```python
from build123d import *

# Parameters (mm, degrees)
F0_W     = 22.349994
F0_H     = 28.762516
F0_R     = 8
F0_R_2   = 2.2479
F1_DEPTH = 3.175
F2_W     = 22.349994
F2_H     = 20.825016
F2_R     = 8
F3_DEPTH = 1.82499
F4_W     = 22.349994
F4_H     = 20.825016
F4_R     = 8
F4_R_2   = 6.412497
F5_DEPTH = 1.5875
F6_R     = 3.96875


with BuildPart() as f1:
    # F0 (on Top) → F1 (new body)
    with BuildSketch(Plane.XY):
        with Locations((0, 14.381258)):
            Rectangle(F0_W, F0_H)
        with Locations((0, 9.650006)):
            Circle(F0_R, mode=Mode.SUBTRACT)
        with Locations((-7.206247, 24.793766)):
            Circle(F0_R_2, mode=Mode.SUBTRACT)
        with Locations((7.206247, 24.793766)):
            Circle(F0_R_2, mode=Mode.SUBTRACT)
    extrude(amount=F1_DEPTH)

    # F2 (on face) → F3 (join)
    with BuildSketch(Plane.XY.offset(3.175)):
        with Locations((0, 10.412508)):
            Rectangle(F2_W, F2_H)
        with Locations((0, 9.650006)):
            Circle(F2_R, mode=Mode.SUBTRACT)
    extrude(amount=F3_DEPTH)

    # F4 (on face) → F5 (join)
    with BuildSketch(Plane.XY.offset(4.99999)):
        with Locations((0, 10.412508)):
            Rectangle(F4_W, F4_H)
        with Locations((0, 9.650006)):
            Circle(F4_R, mode=Mode.SUBTRACT)
        with Locations((0, 9.650006)):
            Circle(F4_R)
        with Locations((0, 9.650006)):
            Circle(F4_R_2, mode=Mode.SUBTRACT)
    extrude(amount=F5_DEPTH)

    # F6
    f6_edges = [f1.edges().sort_by_distance(p)[0] for p in [
        (-11.174997, 28.762516, 1.5875),
    ]]
    fillet(f6_edges, radius=F6_R)


solid = f1.part
```
Check sheet for the modelled part. Datum: model origin and axes. Units: mm. A direction names the side the tool comes from. Give positions to 0.01 mm unless a question says otherwise; leave off trailing zeros. Write each loop counter-clockwise with the first axis right and the second up, starting at its lowest first coordinate (ties: lowest second). Pieces come first, ordered by that corner, then holes. Notation, with made-up numbers: (-4.5, -9) - (-0.5, -9) arc R25 ccw to (-0.5, 29) - close; hole circle Ø4 at (-5, 68). An arc over 180 degrees is marked (long way). Answer as a JSON object with one key per item and string values. Group by question number.
1) Sectioned sample at C-C (z = 1). Give the number of separate pieces and of enclosed holes in the cut face, then the cut area to 3 significant figures.
2) Sectioned sample at B-B (z = 4.5). Record the cut outline in (x, y) (3 decimals), then the cut area to 3 significant figures.
3) Release check for a two-part mould opening along X. For faces 1 (the face through (2.96, 3.96, 5.78)), 2 (the face through (-10.04, 27.57, 1.61)), 3 (the face through (0, 18, 0)) record: pulls with the +X half, pulls with the -X half, needs draft (parallel to the pull), parting line crosses it, or undercut.
4) Access from +Z, -Z, +X, -X, +Y, -Y to the whole of each face (thin tool, end or side, straight path). Record for faces 4 (the face through (6.914, 27.023, 1.565)), 5 (the face through (-1.041, 17.582, 2.465)), 6 (the face through (0, 25, 3.175)).
5) Depth check by flat-ended pin: P1, Ø7, axis at x = -7.21, y = 24.79, coming from the +Z side (3 decimals); P2, Ø8, axis at x = -0.5, y = 11.5, coming from the -Z side; P3, Ø2, axis at x = -7.5, z = 4.5, coming from the +Y side (3 decimals). Enter the tip coordinate at first touch or a pass-through.
6) Sectioned sample at D-D (y = 2.25). Record the cut outline in (x, z) (1 decimal).
7) Thickness scan on probe 1 along Y at (x, z) = (0, 1.5); probe 2 along Y at (x, z) = (-6, 3); probe 3 along Z at (x, y) = (-9.75, 24) (3 decimals). Record the ranges inside material, lowest first. Write a range as from..to.
Geometry results:
{
 "1": {"separate pieces": "1", "enclosed holes": "3", "area": "407 mm^2"},
 "2": {"outline": "(-11.175, 0) - (11.175, 0) - (11.175, 20.825) - (-11.175, 20.825) - close; hole circle Ø16 at (0, 9.65)", "area": "264 mm^2"},
 "3": {"face 1": "undercut", "face 2": "pulls with the -X half", "face 3": "needs draft"},
 "4": {"face 4": "+Z, -Z", "face 5": "-Z", "face 6": "+Z, +X, -X, +Y"},
 "5": {"P1": "stops at z = 3.175", "P2": "passes through", "P3": "stops at y = 20.825"},
 "6": {"outline": "(-11.2, 0) - (-3, 0) - (-3, 5) - (3, 5) - (3, 0) - (11.2, 0) - (11.2, 6.6) - (-11.2, 6.6) - close"},
 "7": {"probe 1": "y = 0..1.65, 17.65..28.76", "probe 2": "y = 0..4.36, 14.94..22.9, 26.69..28.76", "probe 3": "z = 0..3.175"}
}
